Design review of the part built by this model. Coordinates are the model's own, in mm. A direction names the side the tool comes from. Give positions to 0.01 mm unless a question says otherwise; leave off trailing zeros. Order: outer loops, then holes, each group sorted by start corner. A loop starts at its lowest first (then second) coordinate and runs counter-clockwise, first axis right, second up. Notation, with made-up numbers: (64, 2.5) -> (77, 2.5) arc R17 ccw to (77, 25.5) -> close; hole circle Ø3 at (-22, 46.25). An arc over 180 degrees is marked (long way). One line per item, written item: value. Start each with the question number.
1) Consider section D-D (z = 20.25). State the section outline as (x, y) points.
2) Tool access review of faces 4 (the face through (-11.6, -0.5, 9.8)), 5 (the face through (-5.5, -0.5, 8.1)), 6 (the face through (-16.9, 0, 6.3)), 7 (the face through (-17.8, -0.5, 8.1)): name each direction out of +Z, -Z, +X, -X, +Y, -Y from which nothing blocks a thin tool from reaching the whole face with its end or side.
3) The part is to be moulded in two halves that separate along Z. For faces 1 (the face through (-6.3, 0, 6.3)), 2 (the face through (-5.5, -0.5, 4.6)), 3 (the face through (-11.7, -0.5, 3)), say which applies: released by +Z, released by -Z, zero draft, split by the parting line, or undercut.
4) Consider section A-A (x = -11.65). State the section outline as (y, z) points.
5) For pin 1 (0.5 mm diameter, centred on y = -0.5, z = 7.5, fed in from -X); pin 2 (0.6 mm diameter, centred on y = -0.5, z = 6.35, fed in from -X); pin 3 (0.5 mm diameter, centred on x = -10, y = -0.5, fed in from +Z); pin 4 (6 mm diameter, centred on x = -14.5, z = 14.5, fed in from -Y), all flat-tipped, find the tip position at first contact; note any pin that passes through.
6) Wall thickness on line 1 along Z through (x, y) = (-11.65, -0.4); line 2 along Z through (x, y) = (-5.75, -0.5); line 3 along Y through (x, z) = (-2, 3.5): over which ranges is each line inside the solid? List them lowest first. Write a range as from..to.
Autodesk Inventor part; units mm, degrees
ref_plane "YZ Plane" through (0, 0, 0) normal (1, 0, 0) x (0, 1, 0)
ref_plane "XZ Plane" through (0, 0, 0) normal (0, 1, 0) x (-1, 0, 0)
ref_plane "XY Plane" through (0, 0, 0) normal (0, 0, 1) x (1, 0, 0)
sketch "Skizze1" plane through (0, 0, 0) normal (0, 1, 0) x (-1, 0, 0)
  line L0 (0, 0) -> (23.3, 0)
  line L1 (23.3, 0) -> (23.3, 26.8)
  line L2 (23.3, 26.8) -> (0, 26.8)
  line L3 (0, 26.8) -> (0, 0)
  dimension "d0" = 23.3
  dimension "d1" = 26.8
extrude "Extrusion1" add sketch "Skizze1" along normal blind 0.4
sketch "Skizze2" plane through (0, 0, 0) normal (0, -1, 0) x (1, 0, 0)
  line L0 (0, 0) -> (-23.3, 0)
  line L1 (0, 26.8) -> (0, 0)
  line L2 (-23.3, 26.8) -> (0, 26.8)
  line L3 (-23.3, 0) -> (-23.3, 26.8)
  line L4 (-17.8, 3) -> (-5.5, 3)
  line L5 (-5.5, 3) -> (-5.5, 9.8)
  line L6 (-5.5, 9.8) -> (-17.8, 9.8)
  line L7 (-17.8, 9.8) -> (-17.8, 3)
  dimension "d4" = 3
  dimension "d5" = 17
  dimension "d6" = 5.5
  dimension "d7" = 5.5
extrude "Extrusion2" add sketch "Skizze2" along normal blind 1 contours L7 L6 L5 L4
sketch "Skizze3" plane through (0, -1, 0) normal (0, -1, 0) x (1, 0, 0)
  line L0 (-17.8, 3) -> (-5.5, 3)
  line L1 (-5.5, 3) -> (-5.5, 9.8)
  line L2 (-5.5, 9.8) -> (-17.8, 9.8)
  line L3 (-17.8, 9.8) -> (-17.8, 3)
  circle A0 centre (-11.65, 6.4) radius 2.9125
  point P0 (0, 0)
extrude "Extrusion3" cut sketch "Skizze3" against normal through all contours A0
ref_plane "Work Plane1" through (-11.65, 0, 0) normal (-1, 0, 0) x (0, 0, 1)
sketch "Sketch5" plane through (0, 0, 26.8) normal (1, 0, 0) x (0, 0, -1)
  line L0 (23.3125, -1) -> (23.3125, 0.4)
  line L1 (17.4875, -1) -> (17.4875, 0.4)
  circle A0 centre (20.4499, -0.5) radius 0.5025
  point P0 (26.8, 0)
extrude "Extrusion5" cut sketch "Sketch5" against normal through all
ref_plane "Work Plane3" through (-52.1328, -19.1011, -24.6499) normal (0, 1, 0) x (1, 0, 0)
sketch "Sketch6" plane through (-52.1328, -19.1011, -24.6499) normal (0, 1, 0) x (1, 0, 0)
  line L0 (46.6328, -31.0499) -> (52.1328, -31.0499) construction
  line L1 (52.1328, -51.4499) -> (52.1328, -31.0499) construction
  line L2 (28.8328, -51.4499) -> (52.1328, -51.4499) construction
  line L3 (28.8328, -31.0499) -> (28.8328, -51.4499) construction
  line L4 (28.8328, -31.0499) -> (34.3328, -31.0499) construction
  line L5 (34.3328, -31.0499) -> (34.3328, -34.4499) construction
  line L6 (34.3328, -34.4499) -> (46.6328, -34.4499) construction
  line L7 (46.6328, -34.4499) -> (46.6328, -31.0499) construction
  line L8 (6.9828, -36.0499) -> (6.9828, 22.8301) construction
  line L9 (46.6328, -31.5025) -> (34.3328, -31.5025) construction
  line L10 (-16.7355, -31.5025) -> (-33.6581, -41.2728) construction
  line L11 (-33.6581, -41.2728) -> (-33.6581, -21.7322) construction
  line L12 (-33.6581, -21.7322) -> (-16.7355, -31.5025) construction
  point P0 (52.1328, -24.6499)
  point P1 (-28.0172, -31.5025)
  dimension "d16" = 35
hole "Hole1" at (-85.7909, -19.1011, 16.6229) at (-68.8683, -19.1011, 6.8526) at (-85.7909, -19.1011, -2.9177) direction (0, -1, 0) diameter 3.3 depth 12 tip angle 118 counterbore diameter 8 counterbore depth 4
properties part number "02_Nanoscopy_Chip"
Checked values:
1. outline: (-23.3, 0) -> (0, 0) -> (0, 0.4) -> (-23.3, 0.4) -> close
2. face 4: +Z, +X, -X, -Y
2. face 5: +Z, -Z, +X, -Y
2. face 6: +X, -X
2. face 7: +Z, -Z, -X, -Y
3. face 1: undercut
3. face 2: zero draft
3. face 3: released by -Z
4. outline: (-1, 3) -> (0, 3) -> (0, 0) -> (0.4, 0) -> (0.4, 3.49) -> (-1, 3.49) -> close; (-1, 9.31) -> (0.4, 9.31) -> (0.4, 26.8) -> (0, 26.8) -> (0, 9.8) -> (-1, 9.8) -> close
5. pin 1: stops at x = -17.8
5. pin 2: passes through
5. pin 3: stops at z = 9.8
5. pin 4: stops at y = 0
6. line 1: z = 3..3.49, 9.31..9.8
6. line 2: z = 3..5.85, 6.85..9.8
6. line 3: y = 0..0.4
